Build history of the part. All positions in model axes, mm. A direction names the side the tool comes from. Coordinates: 2 decimals unless noted, no trailing zeros. Write each loop counter-clockwise with the first axis right and the second up, starting at its lowest first coordinate (ties: lowest second). Pieces come first, ordered by that corner, then holes.
from build123d import *

# Parameters (mm, degrees)
F0_W     = 64.068158
F0_H     = 53.239739
F1_DEPTH = 84.836
F2_R     = 11.771363
F3_DEPTH = 25.4
F4_W     = 26.12557
F4_H     = 15.822526
F5_DEPTH = 82.55


with BuildPart() as f1:
    # F0 (on Top) → F1 (new body)
    with BuildSketch(Plane.XY):
        with Locations((-5.113421, 3.308685)):
            Rectangle(F0_W, F0_H)
    extrude(amount=F1_DEPTH)

    # F2 (on face) → F3 (join)
    with BuildSketch(Plane.XY.offset(84.836)):
        with Locations((-21.954449, 0)):
            Circle(F2_R)
    extrude(amount=F3_DEPTH)

    # F4 (on face) → F5 (cut)
    with BuildSketch(Plane.XZ.offset(23.311185)):
        with Locations((-2.943726, 56.758301)):
            Rectangle(F4_W, F4_H)
    extrude(amount=-F5_DEPTH, mode=Mode.SUBTRACT)


solid = f1.part
(1) Flat gauge pin, fed straight in: P1, Ø5, axis at x = -3, y = -13, coming from the +Z side. Where does the tip first touch, or does it go through?
(2) Slice it at C-C, the plane y = 22. List the corners of the cut face in (x, z), and give its area (3 significant figures).
(3) 3-axis set-ups, long thin cutter, end or side, ignore diameter. For faces 1 (the cylindrical face through (-10.73, 3.54, 97.36)), 2 (the flat face through (-3, 3, 64.67)), 3 (the flat face through (26.921, 3, 42)): which of +Z, -Z, +X, -X, +Y, -Y reach the whole face in a straight line?
(4) Probe L1, parallel to Z at x = -1, y = 8; L2, parallel to X at y = 9, z = 61; L3, parallel to Z at x = 23, y = -21. List the from-to ranges inside material, lowest first.
(5) Slice it at B-B, the plane z = 58.5. List the corners of the cut face in (x, y), and give its area (3 significant figures).
(6) Slice it at D-D, the plane y = 0. List the corners of the cut face in (x, z), and give its area (3 significant figures).
(7) Two-plate mould, pull along Z, no slides. Class faces 4 (the flat face through (10.119, 3, 57)), 5 (the flat face through (-6, 29.929, 42)), 6 (the flat face through (-22, 0, 110.236)): pulls with the +Z half, pulls with the -Z half, needs draft (parallel to the pull), parting line crosses it, or undercut.
(8) Slice it at A-A, the plane x = -2.5. List the corners of the cut face in (y, z).
Results:
1. P1: stops at z = 84.84
2. outline: (-37.15, 0) - (26.92, 0) - (26.92, 84.84) - (-37.15, 84.84) - close; hole (-16.01, 48.85) - (10.12, 48.85) - (10.12, 64.67) - (-16.01, 64.67) - close
2. area: 5,020 mm2
3. face 1: +Z
3. face 2: +Y, -Y
3. face 3: +Z, -Z, +X, +Y, -Y
4. L1: z = 0 to 48.85, 64.67 to 84.84
4. L2: x = -37.15 to -16.01, 10.12 to 26.92
4. L3: z = 0 to 84.84
5. outline: (-37.15, -23.31) - (-16.01, -23.31) - (-16.01, 29.93) - (-37.15, 29.93) - close; (10.12, -23.31) - (26.92, -23.31) - (26.92, 29.93) - (10.12, 29.93) - close
5. area: 2,020 mm2
6. outline: (-37.15, 0) - (26.92, 0) - (26.92, 84.84) - (-10.18, 84.84) - (-10.18, 110.24) - (-33.73, 110.24) - (-33.73, 84.84) - (-37.15, 84.84) - close; hole (-16.01, 48.85) - (10.12, 48.85) - (10.12, 64.67) - (-16.01, 64.67) - close
6. area: 5,620 mm2
7. face 4: undercut
7. face 5: needs draft
7. face 6: pulls with the +Z half
8. outline: (-23.31, 0) - (29.93, 0) - (29.93, 48.85) - (-23.31, 48.85) - close; (-23.31, 64.67) - (29.93, 64.67) - (29.93, 84.84) - (-23.31, 84.84) - close
